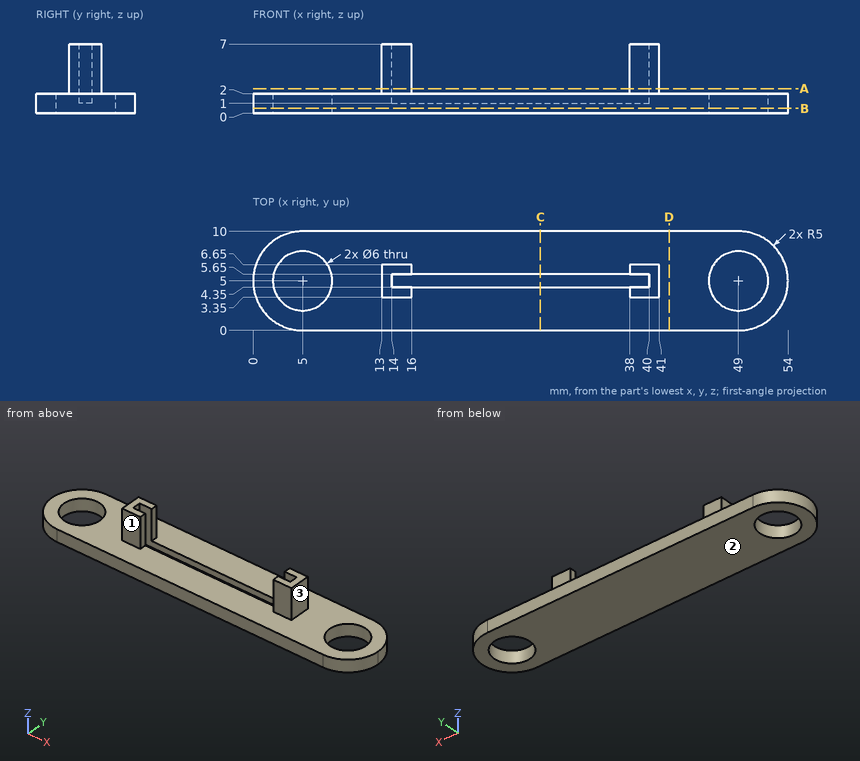
For this review, use the dimensioned drawing (mm, ordinates from the lowest corner) and the shaded views. A direction names the side the tool comes from. Give positions to 0.01 mm unless a question says otherwise; leave off trailing zeros. Order: outer loops, then holes, each group sorted by start corner. A loop starts at its lowest first (then second) coordinate and runs counter-clockwise, first axis right, second up. Notation, with made-up numbers: (-14, 80) - (0, 80) arc R21 ccw to (0, 114) - close; hole circle Ø9 at (40.5, -10.5). An arc over 180 degrees is marked (long way). Use CSV: the item, a comma, the result in double quotes. Start each with the question number.
Q1. For line 1 (Y direction, x = 5, z = 1.3); line 2 (X direction, y = 5.5, z = 0.5); line 3 (Z direction, x = 34, y = 2.75), list the stretches that pass through material, from the lowest coordinate up.
Q2. Take a section at B-B (z = 0.5). State the section outline as (x, y) points.
Q3. Machinability: for the marked faces 1, 2 and 3, which of the approach directions +Z, -Z, +X, -X, +Y, -Y give a long, thin tool a straight path to every point of the face, cutting with its end or side? Answer none if there is none.
Q4. Take a section at D-D (x = 42). State the section outline as (y, z) points, and give its area (3 significant figures).
Q5. Take a section at A-A (z = 2.5). State the section outline as (x, y) points.
Q6. Take a section at C-C (x = 29). State the section outline as (y, z) points.
Q7. For P1, Ø1, axis at x = 29, y = 1.5, coming from the +Z side; P2, Ø1.5, axis at x = 39.5, z = 5.5, coming from the -Y side; P3, Ø4, axis at y = 2, z = 5.5, coming from the -X side, all flat-tipped, find the tip position at first contact; note any pin that passes through.
Calculated:
1,line 1,"y = 0 to 2, 8 to 10"
1,line 2,"x = 0.03 to 2.04, 7.96 to 46.04, 51.96 to 53.97"
1,line 3,"z = 0 to 2"
2,outline,"(5, 0) - (49, 0) arc R5 ccw to (49, 10) - (5, 10) arc R5 ccw to start; hole circle Ø6 at (5, 5); hole circle Ø6 at (49, 5)"
3,face 1,"+Z, +X, -X, -Y"
3,face 2,"-Z, +X, -X, +Y, -Y"
3,face 3,"+Z, +X, +Y, -Y"
4,outline,"(0, 0) - (10, 0) - (10, 2) - (0, 2) - close"
4,area,"20.0 mm²"
5,outline,"(13, 3.35) - (16, 3.35) - (16, 4.35) - (14, 4.35) - (14, 5.65) - (16, 5.65) - (16, 6.65) - (13, 6.65) - close; (38, 3.35) - (41, 3.35) - (41, 6.65) - (38, 6.65) - (38, 5.65) - (40, 5.65) - (40, 4.35) - (38, 4.35) - close"
6,outline,"(0, 0) - (10, 0) - (10, 2) - (5.65, 2) - (5.65, 1) - (4.35, 1) - (4.35, 2) - (0, 2) - close"
7,P1,"stops at z = 2"
7,P2,"stops at y = 3.35"
7,P3,"stops at x = 13"
